Build history of the part. All positions in model axes, mm. Face numbers are marked on the shaded views. Round coordinates to 2 decimals unless told otherwise and drop trailing zeros. Write each loop counter-clockwise with the first axis right and the second up, starting at its lowest first coordinate (ties: lowest second). Pieces come first, ordered by that corner, then holes. Notation, with made-up numbers: (42.5, 4) -> (86.5, 4) arc R6 cw to (86.5, 11) -> close; hole circle Ø7 at (-25.5, 26.5). An arc over 180 degrees is marked (long way). Return JSON: item names as keys, results as strings.
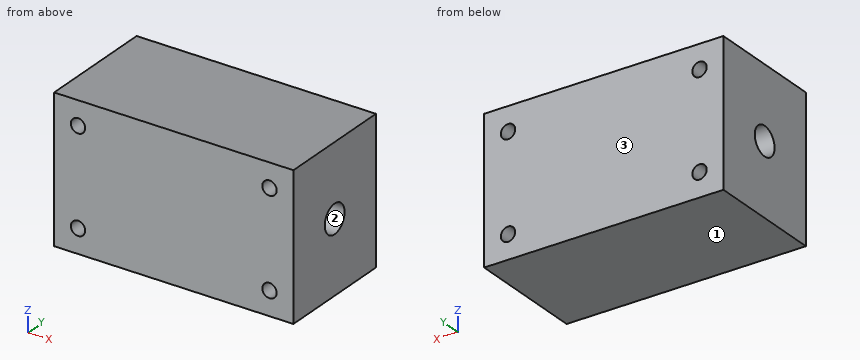
from build123d import *

# Parameters (mm, degrees)
ESQUISSE1_W             = 50
ESQUISSE1_H             = 30
ESQUISSE1_R             = 1.5
BOSS_EXTRU_1_DEPTH      = 25
ENL_V_MAT_EXTRU_1_REACH = 52
ESQUISSE2_R             = 3


with BuildPart() as part:
    # Esquisse1 → Boss.-Extru.1 (new body)
    with BuildSketch(Plane(origin=(0, 0, 0), x_dir=(1, 0, 0), z_dir=(0, 1, 0))):
        Rectangle(ESQUISSE1_W, ESQUISSE1_H)
        with Locations((-20, 10)):
            Circle(ESQUISSE1_R, mode=Mode.SUBTRACT)
        with Locations((-20, -10)):
            Circle(ESQUISSE1_R, mode=Mode.SUBTRACT)
        with Locations((20, -10)):
            Circle(ESQUISSE1_R, mode=Mode.SUBTRACT)
        with Locations((20, 10)):
            Circle(ESQUISSE1_R, mode=Mode.SUBTRACT)
    extrude(amount=BOSS_EXTRU_1_DEPTH)

    # Esquisse2 → Enlèv. mat.-Extru.1 (cut, up to next)
    with BuildSketch(Plane.ZY.offset(25), mode=Mode.PRIVATE) as enl_v_mat_extru_1_sk1:
        with Locations((0, 12.5)):
            Circle(ESQUISSE2_R)
    enl_v_mat_extru_1_tool1 = extrude(enl_v_mat_extru_1_sk1.sketch, amount=-ENL_V_MAT_EXTRU_1_REACH, mode=Mode.PRIVATE) & part.part
    add(enl_v_mat_extru_1_tool1.solids().sort_by_distance((-25, 12.5, 0))[0], mode=Mode.SUBTRACT)


solid = part.part
Q1. Saw through at B-B on x = 20. List the corners of the cut face in (y, z), then the cut area to 3 significant figures.
Verdict:
{"outline": "(0, -15) -> (25, -15) -> (25, -11.5) -> (0, -11.5) -> close; (0, -8.5) -> (25, -8.5) -> (25, 8.5) -> (0, 8.5) -> close; (0, 11.5) -> (25, 11.5) -> (25, 15) -> (0, 15) -> close; hole circle Ø6 at (12.5, 0)", "area": "572 mm²"}
Q2. Wall check: L1, parallel to Z at x = -20, y = 19.25; L2, parallel to Y at x = 8, z = 0.25; L3, parallel to X at y = 8.5, z = -10. Give the ranges that are in metal, low to high.
Verdict:
{"L1": "z = -15 to -11.5, -8.5 to 8.5, 11.5 to 15", "L2": "y = 0 to 9.51, 15.49 to 25", "L3": "x = -25 to -21.5, -18.5 to 18.5, 21.5 to 25"}
Q3. Saw through at C-C on z = -10. List the corners of the cut face in (x, y).
Verdict:
{"outline": "(-25, 0) -> (-21.5, 0) -> (-21.5, 25) -> (-25, 25) -> close; (-18.5, 0) -> (18.5, 0) -> (18.5, 25) -> (-18.5, 25) -> close; (21.5, 0) -> (25, 0) -> (25, 25) -> (21.5, 25) -> close"}
Q4. Saw through at A-A on y = 12.5. List the corners of the cut face in (x, z).
Verdict:
{"outline": "(-25, -15) -> (25, -15) -> (25, -3) -> (-25, -3) -> close; (-25, 3) -> (25, 3) -> (25, 15) -> (-25, 15) -> close; hole circle Ø3 at (-20, -10); hole circle Ø3 at (-20, 10); hole circle Ø3 at (20, -10); hole circle Ø3 at (20, 10)"}
Q5. Saw through at D-D on z = 0. List the corners of the cut face in (x, y).
Verdict:
{"outline": "(-25, 0) -> (25, 0) -> (25, 9.5) -> (-25, 9.5) -> close; (-25, 15.5) -> (25, 15.5) -> (25, 25) -> (-25, 25) -> close"}
Q6. Pin check, flat tips, straight feed: pin 1 Ø5 at (x, z) = (-20, -10) entering from +Y; pin 2 Ø2.5 at (x, z) = (20, -10) entering from -Y. Stop position of each tip, or through.
Verdict:
{"pin 1": "stops at y = 25", "pin 2": "passes through"}
Q7. Two-plate mould, pull along Y, no slides. Class the marked faces 1, 2 and 3: +Y half, -Y half, draft (parallel to the pull), parting line (faces both ways), or undercut.
Verdict:
{"face 1": "draft", "face 2": "undercut", "face 3": "+Y half"}
